```python
from build123d import *

# Parameters (mm, degrees)
SKETCH1_W           = 15
SKETCH1_H           = 3.5
BOSS_EXTRUDE1_DEPTH = 23
SKETCH3_R           = 3
BOSS_EXTRUDE2_DEPTH = 23
SKETCH4_R           = 1.4
CUT_EXTRUDE1_DEPTH  = 23
SKETCH5_R           = 3.5
CUT_EXTRUDE2_DEPTH  = 4.2
SKETCH6_R           = 3.5
CUT_EXTRUDE3_DEPTH  = 4.2
SKETCH7_R           = 4
CUT_EXTRUDE4_DEPTH  = 3
CHAMFER1_SIZE       = 1.5
BOSS_EXTRUDE3_DEPTH = 14.6
FILLET1_R           = 2
FILLET2_R           = 5


with BuildPart() as part:
    # Sketch1 → Boss-Extrude1 (new body)
    with BuildSketch(Plane(origin=(0, 0, 0), x_dir=(1, 0, 0), z_dir=(0, 1, 0))):
        with Locations((-12.213235294, 13.485294118)):
            Rectangle(SKETCH1_W, SKETCH1_H)
        Polygon((-0.713235294, 15.235294118), (-4.713235294, 15.235294118), (-4.713235294, 11.735294118), (-4.713235294, -9.264705882), (-0.713235294, -9.264705882), align=None)
    extrude(amount=BOSS_EXTRUDE1_DEPTH)

    # Sketch3 → Boss-Extrude2 (add)
    with BuildSketch(Plane.XZ):
        with Locations((-2.713235294, 9.264705882)):
            Circle(SKETCH3_R)
    extrude(amount=-BOSS_EXTRUDE2_DEPTH)

    # Sketch4 → Cut-Extrude1 (cut)
    with BuildSketch(Plane.XZ):
        with Locations((-2.713235294, 9.264705882)):
            Circle(SKETCH4_R)
    extrude(amount=-CUT_EXTRUDE1_DEPTH, mode=Mode.SUBTRACT)

    # Sketch5 → Cut-Extrude2 (cut)
    with BuildSketch(Plane.XZ):
        with Locations((-2.713235294, 9.264705882)):
            Circle(SKETCH5_R)
    extrude(amount=-CUT_EXTRUDE2_DEPTH, mode=Mode.SUBTRACT)

    # Sketch6 → Cut-Extrude3 (cut)
    with BuildSketch(Plane(origin=(0, 23, 0), x_dir=(1, 0, 0), z_dir=(0, 1, 0))):
        with Locations((-2.713235294, -9.264705882)):
            Circle(SKETCH6_R)
    extrude(amount=-CUT_EXTRUDE3_DEPTH, mode=Mode.SUBTRACT)

    # Sketch7 → Cut-Extrude4 (cut)
    with BuildSketch(Plane.XY.offset(-11.735294118)):
        with Locations((-13.713235294, 11)):
            Circle(SKETCH7_R)
    extrude(amount=-CUT_EXTRUDE4_DEPTH, mode=Mode.SUBTRACT)

    # Chamfer1
    chamfer1_edges = [part.edges().sort_by_distance(p)[0] for p in [
        (-19.713235294, 11.5, -11.735294118),
    ]]
    chamfer(chamfer1_edges, length=CHAMFER1_SIZE)

    # Sketch8 → Boss-Extrude3 (add)
    with BuildSketch(Plane(origin=(0, 18.8, 0), x_dir=(1, 0, 0), z_dir=(0, 1, 0))):
        Polygon((-0.92234324, -7.637497627), (2.489493511, -7.736371955), (-0.92234324, -3.081041661), align=None)
    extrude(amount=-BOSS_EXTRUDE3_DEPTH)

    # Fillet1
    fillet1_edges = [part.edges().sort_by_distance(p)[0] for p in [
        (-0.713235294, 11.5, -15.235294118),
    ]]
    fillet(fillet1_edges, radius=FILLET1_R)

    # Fillet2
    fillet2_edges = [part.edges().sort_by_distance(p)[0] for p in [
        (-0.713235294, 11.5, 3.36636204),
    ]]
    fillet(fillet2_edges, radius=FILLET2_R)


solid = part.part
```
The listing builds one solid part. Answer for the finished solid, in the listing's coordinates (mm). A direction names the side the tool comes from. Coordinates: 2 decimals unless noted, no trailing zeros. Loops run counter-clockwise (first coordinate to the right, second up) from the corner with the lowest first, then second, coordinate; pieces in that order, holes last. Notation, with made-up numbers: (48, -28) -> (56, -28) arc R15 ccw to (56, -3) -> close; hole circle Ø7 at (-25.75, 28). An arc over 180 degrees is marked (long way). Return JSON: item names as keys, results as strings. Group by question number.
(1) A cutting plane is placed at B-B on z = 3.75. Write down the section's boundary in (x, y), and give its area (3 significant figures).
(2) A cutting plane is placed at C-C on y = 12.75. Write down the section's boundary in (x, z), and give its area (3 significant figures).
(3) A cutting plane is placed at D-D on x = 0.75. Write down the section's boundary in (y, z).
(4) A cutting plane is placed at A-A on y = 8. Write down the section's boundary in (x, z).
(5) Determine the mould class of faces 5 (the flat face through (-0.713, 11, -3)), 6 (the flat face through (-14, 11, -14.735)), 7 (the flat face through (-19.713, 11, -14)) for opening direction X: released by +X, released by -X, zero draft, split by the parting line, or undercut.
(6) Which of the six approach directions +Z, -Z, +X, -X, +Y, -Y give full straight-line access (tool end or side, diameter ignored) to faces 1 (the cylindrical face through (-2.683, 20.929, 5.765)), 2 (the flat face through (-4.713, 11, -2)), 3 (the cylindrical face through (-9.898, 12.201, -13.214)), 4 (the cylindrical face through (-2.743, 2.071, 5.765))?
(7) Given pin 1 Ø11 at (x, y) = (-10.5, 8) entering from +Z; pin 2 Ø8 at (y, z) = (15.5, 5) entering from +X; pin 3 Ø4 at (y, z) = (15, 1.5) entering from +X; pin 4 Ø10 at (x, z) = (-14, 7.5) entering from -Y, each flat-ended and moving along its own axis, determine where each tip first touches the part or whether it passes through.
(8) Find the intervals of material crossed by probe 1 along Z at (x, y) = (-11.25, 2); probe 2 along Z at (x, y) = (-11.5, 12.75); probe 3 along X at (y, z) = (1.5, 2.75), in increasing order. Write a range as from..to.
The answers:
{
 "1": {"outline": "(-4.71, 0) -> (-0.71, 0) -> (-0.71, 4.2) -> (-0.29, 4.2) -> (-0.29, 18.8) -> (-0.71, 18.8) -> (-0.71, 23) -> (-4.71, 23) -> close", "area": "98.2 mm^2"},
 "2": {"outline": "(-19.71, -15.24) -> (-2.71, -15.24) arc R2 ccw to (-0.71, -13.24) -> (-0.71, 1.73) arc R5 cw to (0.25, 4.69) -> (2.49, 7.74) -> (-0.18, 7.66) arc R3 ccw (long way) to (-4.71, 7.03) -> (-4.71, -11.74) -> (-10.12, -11.74) -> (-10.12, -14.74) -> (-17.31, -14.74) -> (-17.31, -11.74) -> (-18.21, -11.74) -> (-19.71, -13.24) -> close; hole circle Ø2.8 at (-2.71, 9.26)", "area": "145 mm^2"},
 "3": {"outline": "(4.2, 5.36) -> (18.8, 5.36) -> (18.8, 7.69) -> (4.2, 7.69) -> close"},
 "4": {"outline": "(-19.71, -15.24) -> (-2.71, -15.24) arc R2 ccw to (-0.71, -13.24) -> (-0.71, 1.73) arc R5 cw to (0.25, 4.69) -> (2.49, 7.74) -> (-0.18, 7.66) arc R3 ccw (long way) to (-4.71, 7.03) -> (-4.71, -11.74) -> (-11.07, -11.74) -> (-11.07, -14.74) -> (-16.36, -14.74) -> (-16.36, -11.74) -> (-18.21, -11.74) -> (-19.71, -13.24) -> close; hole circle Ø2.8 at (-2.71, 9.26)"},
 "5": {"face 5": "released by +X", "face 6": "undercut", "face 7": "released by -X"},
 "6": {"face 1": "+Z, +Y", "face 2": "-X, +Y, -Y", "face 3": "+Z", "face 4": "+Z, -Y"},
 "7": {"pin 1": "stops at z = 11.21", "pin 2": "stops at x = 2.49", "pin 3": "stops at x = -0.39", "pin 4": "passes through"},
 "8": {"probe 1": "z = -15.24..-11.74", "probe 2": "z = -15.24..-14.74", "probe 3": "x = -4.71..-0.71"}
}
